Work out the finished part from the listing and answer in its coordinate system (mm). Coordinates: 2 decimals unless noted, no trailing zeros. Order: outer loops, then holes, each group sorted by start corner. A loop starts at its lowest first (then second) coordinate and runs counter-clockwise, first axis right, second up. Notation, with made-up numbers: (61.25, 44.25) - (109.25, 44.25) arc R17 ccw to (109.25, 52.25) - close; hole circle Ø10 at (0.5, 61). An arc over 180 degrees is marked (long way). Answer as a JSON object with one key per item and string values. Group by question number.
1) Section A-A (y = -5) is taken. Give the vertices of the cut face in (x, z), plus the area to 3 significant figures.
2) Each of these flat-tipped pins is pushed along its axis until it touches: P1, Ø3.5, axis at x = -8, y = -5, coming from the +Z side; P2, Ø2, axis at x = -7.5, y = -4.5, coming from the -Z side; P3, Ø3.5, axis at x = 272.5, z = 53.61, coming from the -Y side. Where does it stop, or does it pass through?
3) Find the intervals of material crossed by line 1 along Z through (x, y) = (-272.5, -2.75); line 2 along X through (y, z) = (-5, 7.25); line 3 along X through (y, z) = (-3, 48.5), in increasing order.
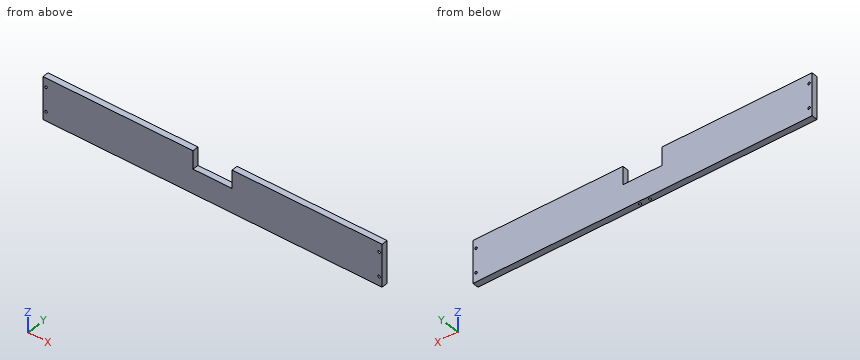
from build123d import *

# Parameters (mm, degrees)
F0_R     = 2
F1_DEPTH = 10
F2_R     = 2
F3_DEPTH = 15


with BuildPart() as f1:
    # F0 (on Front) → F1 (new body)
    with BuildSketch(Plane.XZ):
        Polygon((-32, 68.609319), (-277.5, 68.609319), (-277.5, -1.390681), (277.5, -1.390681), (277.5, 68.609319), (32, 68.609319), (32, 38.609319), (0, 38.609319), (-32, 38.609319), align=None)
        with Locations((-272.5, 13.609319)):
            Circle(F0_R, mode=Mode.SUBTRACT)
        with Locations((272.5, 13.609319)):
            Circle(F0_R, mode=Mode.SUBTRACT)
        with Locations((-272.5, 53.609319)):
            Circle(F0_R, mode=Mode.SUBTRACT)
        with Locations((272.5, 53.609319)):
            Circle(F0_R, mode=Mode.SUBTRACT)
    extrude(amount=F1_DEPTH)

    # F2 (on face) → F3 (cut)
    with BuildSketch(Plane(origin=(0, 0, -1.390681), x_dir=(1, 0, 0), z_dir=(0, 0, -1))):
        with Locations((-8, 5)):
            Circle(F2_R)
        with Locations((8, 5)):
            Circle(F2_R)
    extrude(amount=-F3_DEPTH, mode=Mode.SUBTRACT)


solid = f1.part
Report:
{
 "1": {"outline": "(-277.5, -1.39) - (-10, -1.39) - (-10, 13.61) - (-6, 13.61) - (-6, -1.39) - (6, -1.39) - (6, 13.61) - (10, 13.61) - (10, -1.39) - (277.5, -1.39) - (277.5, 68.61) - (32, 68.61) - (32, 38.61) - (-32, 38.61) - (-32, 68.61) - (-277.5, 68.61) - close; hole circle Ø4 at (-272.5, 13.61); hole circle Ø4 at (-272.5, 53.61); hole circle Ø4 at (272.5, 13.61); hole circle Ø4 at (272.5, 53.61)", "area": "36,800 mm²"},
 "2": {"P1": "stops at z = 38.61", "P2": "stops at z = 13.61", "P3": "passes through"},
 "3": {"line 1": "z = -1.39 to 11.61, 15.61 to 51.61, 55.61 to 68.61", "line 2": "x = -277.5 to -10, -6 to 6, 10 to 277.5", "line 3": "x = -277.5 to -32, 32 to 277.5"}
}
